Read the model definition and answer for the solid it produces. Units are mm, in the model's axes. A direction names the side the tool comes from. Give positions to 0.01 mm unless a question says otherwise; leave off trailing zeros. Loops run counter-clockwise (first coordinate to the right, second up) from the corner with the lowest first, then second, coordinate; pieces in that order, holes last. Notation, with made-up numbers: (57, 59) - (78, 59) arc R21 cw to (78, 79) - close; hole circle Ø5 at (38.5, 5). An arc over 180 degrees is marked (long way). Put each result on its own line as item: value. Start each with the question number.
1. Given pin 1 Ø1.8 at (x, z) = (-22.25, -17.5) entering from -Y; pin 2 Ø0.8 at (x, y) = (28, 1) entering from -Z, each flat-ended and moving along its own axis, determine where each tip first touches the part or whether it passes through.
2. A cutting plane is placed at A-A, the plane z = -17.5. Determine the outline of the cut face in (x, y), plus the area to 3 significant figures.
3. For faces 1 (the flat face through (-26.5, 1, 0)), 2 (the flat face through (-28, 1, -10)), 3 (the flat face through (25, 1, -15)), determine the directions among +Z, -Z, +X, -X, +Y, -Y from which every point of the face is accessible in a straight line to the end or side of a thin tool.
4. For a pull along X with two mould halves and no side action, classify faces 4 (the flat face through (28, 1, -10)), 5 (the flat face through (27, 1, -5)), 6 (the flat face through (28, 1, 0)), 7 (the flat face through (-25, 1, -15)) as released by +X, released by -X, zero draft, split by the parting line, or undercut.
5. A cutting plane is placed at D-D, the plane y = 1.1. Determine the outline of the cut face in (x, z), plus the area to 3 significant figures.
6. A cutting plane is placed at B-B, the plane x = -22.25. Determine the outline of the cut face in (y, z).
7. Consider L1, parallel to Z at x = -22.25, y = 0.75; L2, parallel to X at y = 1.25, z = 1; L3, parallel to X at y = 0.5, z = -17.5. Determine where each line is inside the solid, lowest interval first. Write a range as from..to.
8. A cutting plane is placed at C-C, the plane z = 13. Determine the outline of the cut face in (x, y), plus the area to 3 significant figures.
Autodesk Inventor part; units mm, degrees
ref_plane "Work Plane1" through (0, 0, 10) normal (-1, 0, 0) x (0, 0, 1)
ref_plane "Work Plane2" through (25, 0, 0) normal (0, 0, -1) x (-1, 0, 0)
ref_plane "YZ Plane" through (0, 0, 0) normal (1, 0, 0) x (0, 1, 0)
sketch "Sketch1" plane through (0, 0, 0) normal (0, 1, 0) x (-1, 0, 0)
  circle A0 centre (0, 0) radius 8.5
  line L0 (19.5, 15) -> (-19.5, 15)
  line L1 (-19.5, 15) -> (-19.5, -15)
  line L2 (-19.5, -15) -> (19.5, -15)
  line L3 (19.5, -15) -> (19.5, 15)
  line L4 (19.5, 15) -> (-19.5, -15) construction
  line L5 (-19.5, 15) -> (19.5, -15) construction
  line L6 (25, 20) -> (-25, 20)
  line L7 (-25, 20) -> (-25, -20)
  line L8 (-25, -20) -> (25, -20)
  line L9 (25, -20) -> (25, 20)
  line L10 (25, 20) -> (-25, -20) construction
  line L11 (-25, 20) -> (25, -20) construction
  line L12 (-25, 0) -> (-30, 0)
  line L13 (-30, 0) -> (-30, -10)
  line L14 (-30, -10) -> (-25, -10)
  line L15 (-25, -10) -> (-25, 0)
  line L16 (-30, 0) -> (-25, 0)
  line L17 (-25, 0) -> (-25, 10)
  line L18 (-25, 10) -> (-30, 10)
  line L19 (-30, 10) -> (-30, 0)
  line L20 (-25, 10) -> (-25, 5)
  line L21 (-25, 5) -> (-26.5, 5)
  line L22 (-26.5, 5) -> (-28, 5)
  line L23 (-28, 5) -> (-28, -5)
  line L24 (-28, -5) -> (-26.5, -5)
  line L25 (-26.5, -5) -> (-26.5, 5)
  line L26 (0, 0) -> (0, -20)
  line L27 (30, 0) -> (30, -10)
  line L28 (30, -10) -> (25, -10)
  line L29 (25, 10) -> (30, 10)
  line L30 (30, 10) -> (30, 0)
  line L31 (26.5, 5) -> (28, 5)
  line L32 (28, 5) -> (28, -5)
  line L33 (28, -5) -> (26.5, -5)
  line L34 (26.5, -5) -> (26.5, 5)
  dimension "d0" = 17
  dimension "d1" = 39
  dimension "d2" = 30
  dimension "d3" = 50
  dimension "d4" = 40
  dimension "d5" = 5
  dimension "d6" = 10
  dimension "d7" = 5
  dimension "d8" = 10
  dimension "d9" = 5
  dimension "d10" = 1.5
  dimension "d11" = 1.5
  dimension "d12" = 10
extrude "Extrusion1" add sketch "Sketch1" along normal blind 1.5 contours L8 L7 L6 L9 | L14 L13 L12 L23 L24 L25 L7 | L9 L29 L30 L27 L28 | L12 L25 L21 L7 | L21 L22 L23 L12 L19 L18 L7
sketch "Sketch2" plane through (0, 1.5, 0) normal (0, 1, 0) x (1, 0, 0)
  line L0 (19.5, -15) -> (-19.5, -15)
  line L1 (-19.5, -15) -> (-22.25, -15)
  line L2 (-22.25, -15) -> (-22.25, -17.5)
  line L3 (-25, -20) -> (25, -20)
  circle A0 centre (-22.25, -17.5) radius 1.5
  point P0 (0, 0)
  dimension "d15" = 2.75
  dimension "d16" = 2.5
  dimension "d17" = 3
extrude "Extrusion2" cut sketch "Sketch2" against normal blind 1.5
ref_plane "Work Plane1" through (0, 0, 10) normal (-1, 0, 0) x (0, 0, 1)
ref_plane "Work Plane2" through (25, 0, 0) normal (0, 0, -1) x (-1, 0, 0)
mirror "Mirror1" about plane through (0, 0, 10) normal (-1, 0, 0) of "Extrusion2"
mirror "Mirror2" about plane through (25, 0, 0) normal (0, 0, -1) of "Extrusion2", "Mirror1"
ref_plane "Work Plane3" through (0, 0, 10) normal (-1, 0, 0) x (0, 0, 1)
ref_plane "Work Plane4" through (0, 0, -10) normal (1, 0, 0) x (0, 0, -1)
ref_plane "Work Plane5" through (0, 0, -10) normal (1, 0, 0) x (0, 0, -1)
properties part number "topBearingHolder"
Return value:
1. pin 1: passes through
1. pin 2: stops at z = -10
2. outline: (-25, 0) - (-23.75, 0) - (-23.75, 1.5) - (-25, 1.5) - close; (-20.75, 0) - (20.75, 0) - (20.75, 1.5) - (-20.75, 1.5) - close; (23.75, 0) - (25, 0) - (25, 1.5) - (23.75, 1.5) - close
2. area: 66.0 mm2
3. face 1: +Y, -Y
3. face 2: -Z, -X, +Y, -Y
3. face 3: -Z, +X, +Y, -Y
4. face 4: zero draft
4. face 5: undercut
4. face 6: undercut
4. face 7: released by -X
5. outline: (-30, -10) - (-25, -10) - (-25, -20) - (25, -20) - (25, -10) - (30, -10) - (30, 10) - (25, 10) - (25, 20) - (-25, 20) - (-25, 10) - (-30, 10) - close; hole (-28, -5) - (-26.5, -5) - (-26.5, 5) - (-28, 5) - close; hole circle Ø3 at (-22.25, -17.5); hole circle Ø3 at (-22.25, 17.5); hole (-19.5, -15) - (19.5, -15) - (19.5, 15) - (-19.5, 15) - close; hole circle Ø3 at (22.25, -17.5); hole circle Ø3 at (22.25, 17.5); hole (26.5, -5) - (28, -5) - (28, 5) - (26.5, 5) - close
5. area: 972 mm2
6. outline: (0, -20) - (1.5, -20) - (1.5, -19) - (0, -19) - close; (0, -16) - (1.5, -16) - (1.5, 16) - (0, 16) - close; (0, 19) - (1.5, 19) - (1.5, 20) - (0, 20) - close
7. L1: z = -20..-19, -16..16, 19..20
7. L2: x = -30..-28, -26.5..-19.5, 19.5..26.5, 28..30
7. L3: x = -25..-23.75, -20.75..20.75, 23.75..25
8. outline: (-25, 0) - (-19.5, 0) - (-19.5, 1.5) - (-25, 1.5) - close; (19.5, 0) - (25, 0) - (25, 1.5) - (19.5, 1.5) - close
8. area: 16.5 mm2
